Can you work these out from the model? Positions are in its coordinate system, mm. Face numbers are marked on the shaded views. Coordinates: 2 decimals unless noted, no trailing zeros. Order: outer loops, then holes, each group sorted by start corner. A loop starts at its lowest first (then second) coordinate and runs counter-clockwise, first axis right, second up. Notation, with made-up numbers: (65, 46) - (109, 46) arc R29 cw to (109, 84) - close; hole circle Ø2 at (39.5, 2.5). An arc over 180 degrees is marked (long way). Return JSON: item names as keys, results as strings. Group by question number.
1) Imagine slicing it at C-C (z = 13). Write out the boundary of the cut face in (x, y), and give its area (3 significant figures).
2) For pin 1 Ø12 at (x, y) = (3, -16) entering from +Z; pin 2 Ø1.5 at (x, y) = (-9, 6) entering from -Z; pin 3 Ø6 at (x, y) = (-5, -11.5) entering from +Z; pin 4 Ø8 at (y, z) = (23, -25) entering from -X, each with a flat end and sliding along its axis, tell me the tip position at first contact or that it passes through.
3) Imagine slicing it at B-B (x = 3). Write out the boundary of the cut face in (y, z), and give its area (3 significant figures).
4) If we mould it in two halves opening along Y, with no side actions, what happens to the marked faces 1 and 2? For each: pulls with the +Y half, pulls with the -Y half, needs draft (parallel to the pull), parting line crosses it, or undercut.
5) Imagine slicing it at A-A (z = -3.5). Write out the boundary of the cut face in (x, y).
6) If I drill on line 1 along X through (y, z) = (-5, 18); line 2 along Z through (x, y) = (15.5, 4); line 3 along Y through (x, z) = (-4, 14), over which ranges is the centre line in solid material (lowest first)?
```python
from build123d import *

# Parameters (mm, degrees)
SKETCH1_R           = 5.08
BOSS_EXTRUDE1_DEPTH = 17.78
SKETCH2_R           = 31.75
BOSS_EXTRUDE2_DEPTH = 12.7
CUT_EXTRUDE2_DEPTH  = 49.293409488
CIRPATTERN2_COUNT   = 30


with BuildPart() as part:
    # Sketch1 → Boss-Extrude1 (new body)
    with BuildSketch(Plane(origin=(0, 0, 0), x_dir=(0, 0, -1), z_dir=(1, 0, 0))):
        Circle(SKETCH1_R)
    extrude(amount=BOSS_EXTRUDE1_DEPTH)

    # Sketch2 → Boss-Extrude2 (add)
    with BuildSketch(Plane.ZY):
        Circle(SKETCH2_R)
    extrude(amount=BOSS_EXTRUDE2_DEPTH)

    # Sketch5 → Cut-Extrude2 (cut, through all)
    with BuildSketch(Plane(origin=(0, 0, 0), x_dir=(0, 0, -1), z_dir=(1, 0, 0))):
        with BuildLine():
            Line((0, 29.980101005), (1.723107067, 31.703208072))
            ThreePointArc((1.723107067, 31.703208072), (0, 31.75), (-1.723107067, 31.703208072))
            Line((-1.723107067, 31.703208072), (0, 29.980101005))
        make_face()
    cut_extrude2 = extrude(amount=-CUT_EXTRUDE2_DEPTH, mode=Mode.SUBTRACT)

    # CirPattern2: Cut-Extrude2 ×30 about axis
    cirpattern2_axis = Axis((0, 0, 0), (1, 0, 0))
    for i in range(1, CIRPATTERN2_COUNT):
        add(cut_extrude2.rotate(cirpattern2_axis, i * 360 / CIRPATTERN2_COUNT), mode=Mode.SUBTRACT)


solid = part.part
```
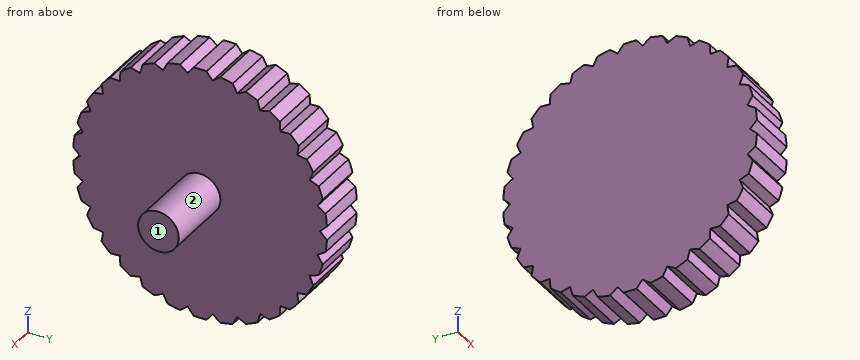
Calculated:
{
 "1": {"outline": "(-12.7, -27.7) - (0, -27.7) - (0, 27.7) - (-12.7, 27.7) - close", "area": "704 mm2"},
 "2": {"pin 1": "z = 29.62", "pin 2": "z = -31.31", "pin 3": "z = 30.01", "pin 4": "x = -12.7"},
 "3": {"outline": "circle Ø10.16 at (0, 0)", "area": "81.1 mm2"},
 "4": {"face 1": "needs draft", "face 2": "parting line crosses it"},
 "5": {"outline": "(-12.7, -31.56) - (0, -31.56) - (0, -3.68) - (17.78, -3.68) - (17.78, 3.68) - (0, 3.68) - (0, 31.56) - (-12.7, 31.56) - close"},
 "6": {"line 1": "-12.7 to 0", "line 2": "-3.13 to 3.13", "line 3": "-28.08 to 28.08"}
}
